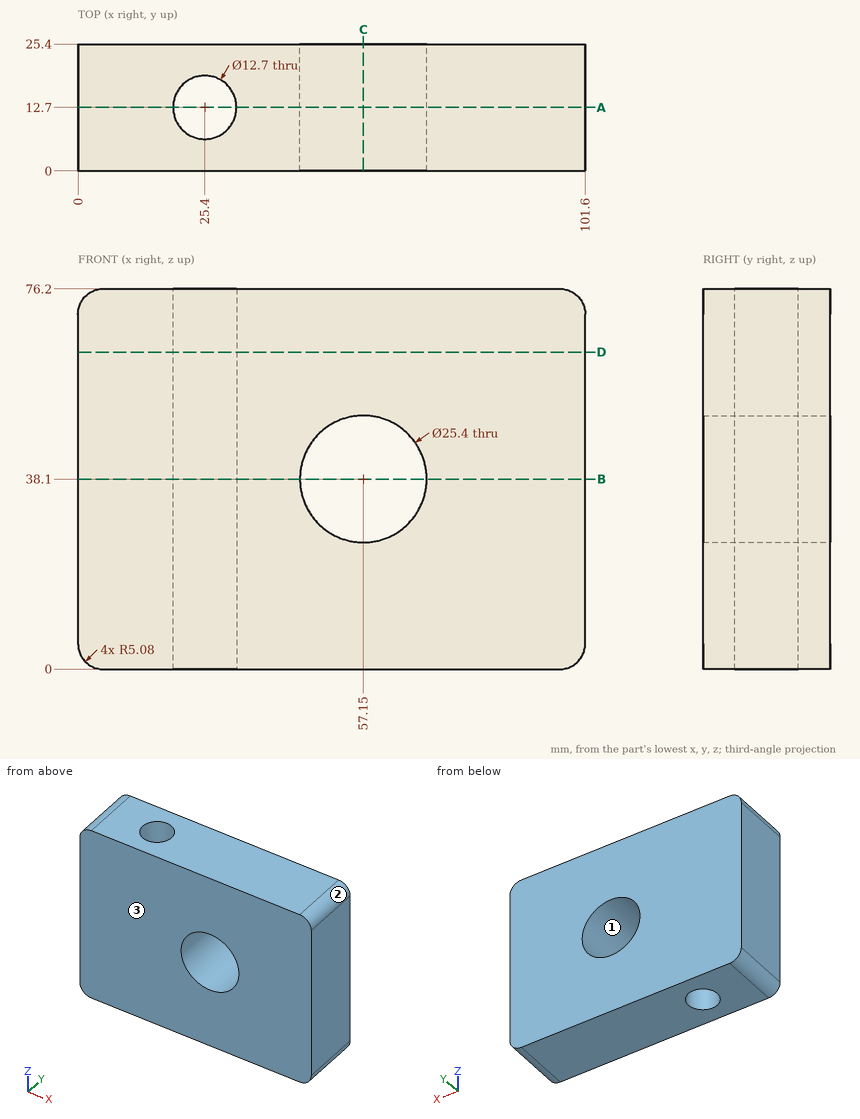
Geometry: see drawing. Coordinates: mm, zero at the bounding-box minimum. Coordinates: 2 decimals unless noted, no trailing zeros. Write each loop counter-clockwise with the first axis right and the second up, starting at its lowest first coordinate (ties: lowest second). Pieces come first, ordered by that corner, then holes.
1) Mould query, pull axis Z, two halves, no side actions, for the marked faces 1, 2 and 3. Classes: pulls with the +Z half, pulls with the -Z half, needs draft (parallel to the pull), parting line crosses it, or undercut.
2) Material intervals for line 1 along Y through (x, z) = (25, 46); line 2 along Z through (x, y) = (57.15, 19.25); line 3 along X through (y, z) = (13, 17.5), sorted ascending.
3) Section A-A on y = 12.7. Output: boundary loops of the cut face in (x, z).
4) Section B-B on z = 38.1. Output: boundary loops of the cut face in (x, y).
5) Section C-C on x = 57.15. Output: boundary loops of the cut face in (y, z).
6) Section D-D on z = 63.5. Output: boundary loops of the cut face in (x, y), and give its area (3 significant figures).
Check result:
1. face 1: undercut
1. face 2: pulls with the +Z half
1. face 3: needs draft
2. line 1: y = 0 to 6.36, 19.04 to 25.4
2. line 2: z = 0 to 25.4, 50.8 to 76.2
2. line 3: x = 0 to 19.06, 31.74 to 101.6
3. outline: (0, 5.08) arc R5.08 ccw to (5.08, 0) - (19.05, 0) - (19.05, 76.2) - (5.08, 76.2) arc R5.08 ccw to (0, 71.12) - close; (31.75, 0) - (96.52, 0) arc R5.08 ccw to (101.6, 5.08) - (101.6, 71.12) arc R5.08 ccw to (96.52, 76.2) - (31.75, 76.2) - close; hole circle Ø25.4 at (57.15, 38.1)
4. outline: (0, 0) - (44.45, 0) - (44.45, 25.4) - (0, 25.4) - close; (69.85, 0) - (101.6, 0) - (101.6, 25.4) - (69.85, 25.4) - close; hole circle Ø12.7 at (25.4, 12.7)
5. outline: (0, 0) - (25.4, 0) - (25.4, 25.4) - (0, 25.4) - close; (0, 50.8) - (25.4, 50.8) - (25.4, 76.2) - (0, 76.2) - close
6. outline: (0, 0) - (101.6, 0) - (101.6, 25.4) - (0, 25.4) - close; hole circle Ø12.7 at (25.4, 12.7)
6. area: 2,450 mm2
